from build123d import *

# Parameters (mm, degrees)
SKETCH_1_W                   = 25
SKETCH_1_H                   = 25
SKETCH_1_R                   = 1.5
EXTRUDE_1_DEPTH              = 7.65
SKETCH_2_R                   = 1.51
EXTRUDE_2_DEPTH              = 3
SKETCH_3_R                   = 7.5
CUT_EXTRUDE_1_DEPTH          = 5
SKETCH_4_R                   = 2.8
CUT_EXTRUDE_2_DEPTH          = 2
SKETCH_5_R                   = 1.55
CUT_EXTRUDE_3_DEPTH          = 2
SKETCH_6_W                   = 7.593154143
SKETCH_6_H                   = 30.65177665
CUT_EXTRUDE_4_DEPTH          = 30.911076544
EXTRUDE_START                = 0.5
SKETCH_7_R                   = 10
SKETCH_7_R_2                 = 7.5
EXTRUDE_3_DEPTH              = 0.5
FILLET_4_R                   = 2
HOLE_WIZARD_M2_1_D           = 1.6
HOLE_WIZARD_M2_1_CSINK_D     = 2.05
HOLE_WIZARD_M2_1_CSINK_ANGLE = 90


with BuildPart() as part:
    # 草图1 → 凸台-拉伸1 (new body)
    # profile 1 of 2: a face of its own
    with BuildSketch(Plane.XY):
        Rectangle(SKETCH_1_W, SKETCH_1_H)
        Circle(SKETCH_1_R, mode=Mode.SUBTRACT)
    # profile 2 of 2: a face of its own
    with BuildSketch(Plane.XY):
        Circle(SKETCH_1_R)
    extrude(amount=EXTRUDE_1_DEPTH)

    # 草图2 → 凸台-拉伸2 (add)
    with BuildSketch(Plane.XY.offset(7.65)):
        Circle(SKETCH_2_R)
    extrude(amount=EXTRUDE_2_DEPTH)

    # 草图3 → 切除-拉伸1 (cut)
    with BuildSketch(Plane(origin=(0, 0, 0), x_dir=(-1, 0, 0), z_dir=(0, 0, -1))):
        Circle(SKETCH_3_R)
    extrude(amount=-CUT_EXTRUDE_1_DEPTH, mode=Mode.SUBTRACT)

    # 草图4 → 切除-拉伸2 (cut)
    with BuildSketch(Plane.XY.offset(7.65)):
        with Locations((4.5, 0)):
            Circle(SKETCH_4_R)
        with Locations((-4.5, 0)):
            Circle(SKETCH_4_R)
    extrude(amount=-CUT_EXTRUDE_2_DEPTH, mode=Mode.SUBTRACT)

    # 草图5 → 切除-拉伸3 (cut)
    with BuildSketch(Plane.XY.offset(5.65)):
        with Locations((4.5, 0)):
            Circle(SKETCH_5_R)
        with Locations((-4.5, 0)):
            Circle(SKETCH_5_R)
    extrude(amount=-CUT_EXTRUDE_3_DEPTH, mode=Mode.SUBTRACT)

    # 草图6 → 切除-拉伸4 (cut, through all)
    with BuildSketch(Plane.ZY.offset(12.5)):
        with Locations((-2.946577072, 0.223328063)):
            Rectangle(SKETCH_6_W, SKETCH_6_H)
    extrude(amount=-CUT_EXTRUDE_4_DEPTH, mode=Mode.SUBTRACT)

    # 草图7 → 凸台-拉伸3 (add)
    with BuildSketch(Plane(origin=(0, 0, 0.85), x_dir=(-1, 0, 0), z_dir=(0, 0, -1)).offset(EXTRUDE_START)):
        with Locations(Location((0, 0, 0), (0, 0, 90))):
            Circle(SKETCH_7_R)
        Circle(SKETCH_7_R_2, mode=Mode.SUBTRACT)
    extrude(amount=-EXTRUDE_3_DEPTH)

    # 圆角4
    # the kernel refuses this fillet: 2 mm, written as the material it adds along each edge
    with BuildSketch(Plane(origin=(0, 0, 0.85), x_dir=(0, 1, 0), z_dir=(-1, 0, 0))) as fillet_4_piece_1:
        with BuildLine():
            CenterArc((11.322875656, 2), FILLET_4_R, 228.590377891, 41.409622109)
            Line((11.322875656, 0), (11.322875656, -0.04))
            Line((11.322875656, -0.04), (10, -0.04))
            Line((10, -0.04), (9.96, 0))
            ThreePointArc((9.96, 0), (9.96, 0.25), (9.973542487, 0.47))
            Line((9.973542487, 0.47), (10, 0.5))
        make_face()
    revolve(axis=Axis((0, 0, 0.85), (0, 0, -1)))

    # M2 螺纹孔1 (through all)
    with Locations(Plane.XY.offset(7.65)):
        with Locations((-10, 10), (10, 10), (-10, -10), (10, -10)):
            CounterSinkHole(HOLE_WIZARD_M2_1_D / 2, HOLE_WIZARD_M2_1_CSINK_D / 2, counter_sink_angle=HOLE_WIZARD_M2_1_CSINK_ANGLE)


solid = part.part
Read the model definition and answer for the solid it produces. Units are mm, in the model's axes. A direction names the side the tool comes from. Give positions to 0.01 mm unless a question says otherwise; leave off trailing zeros. Write each loop counter-clockwise with the first axis right and the second up, starting at its lowest first coordinate (ties: lowest second). Pieces come first, ordered by that corner, then holes. Notation, with made-up numbers: (71, 78) - (76, 78) arc R35 cw to (76, 111) - close; hole circle Ø7 at (-39.5, 37). An arc over 180 degrees is marked (long way). Use CSV: the item, a comma, the result in double quotes. Start each with the question number.
Item 1: Consider line 1 (Y direction, x = -10, z = 3.75); line 2 (X direction, y = -1.5, z = 6.5). Determine where each line is inside the solid, lowest interval first.
Item 2: The part is cut by section A-A, the plane x = 0. Give the vertices of the cut face in (y, z).
Item 3: The mould has two halves that part along Y. Classify faces 4 (the cylindrical face through (-0.197, 1.497, 9.129)), 5 (the flat face through (0, 12.5, 4)), 6 (the cylindrical face through (-9.896, -9.207, 4.091)): pulls with the +Y half, pulls with the -Y half, needs draft (parallel to the pull), parting line crosses it, or undercut.
Item 4: The part is cut by section C-C, the plane y = -0.5. Count the separate pieces of the cut face and the enclosed holes in it, and give its area (3 significant figures).
Item 5: The part is cut by section B-B, the plane z = 1.5. Give the vertices of the cut face in (x, y).
Item 6: Flat-ended cylindrical pins translate along their axes: P1, Ø4, axis at x = -4.5, y = 0, coming from the +Z side; P2, Ø10, axis at x = 5, y = -6.5, coming from the +Z side; P3, Ø5, axis at x = 4.5, y = 0, coming from the -Z side; P4, Ø1, axis at x = 10, y = -10, coming from the -Z side. Find the tip coordinate at first contact, or state that the pin passes through.
Item 7: For faces 1 (the flat face through (-12.5, 0, 4)), 2 (the flat face through (0, 0, 5)), 3 (the flat face through (6, -1, 5.65)), determine the directions among +Z, -Z, +X, -X, +Y, -Y from which every point of the face is accessible in a straight line to the end or side of a thin tool.
Item 8: The part is cut by section D-D, the plane z = 9. Give the vertices of the cut face in (x, y).
Taken from the geometry:
1,line 1,"-12.5 to -10.8, -9.2 to 9.2, 10.8 to 12.5"
1,line 2,"-12.5 to -6.86, -2.14 to 2.14, 6.86 to 12.5"
2,outline,"(-12.5, 0.85) - (-11.32, 0.85) arc R2 cw to (-10, 0.35) - (-7.5, 0.35) - (-7.5, 5) - (7.5, 5) - (7.5, 0.35) - (10, 0.35) arc R2 cw to (11.32, 0.85) - (12.5, 0.85) - (12.5, 7.65) - (1.51, 7.65) - (1.51, 10.65) - (-1.51, 10.65) - (-1.51, 7.65) - (-12.5, 7.65) - close"
3,face 4,"parting line crosses it"
3,face 5,"pulls with the +Y half"
3,face 6,"undercut"
4,separate pieces,"3"
4,enclosed holes,"0"
4,area,"93.5 mm2"
5,outline,"(-12.5, -12.5) - (12.5, -12.5) - (12.5, 12.5) - (-12.5, 12.5) - close; hole circle Ø1.6 at (-10, -10); hole circle Ø1.6 at (-10, 10); hole circle Ø15 at (0, 0); hole circle Ø1.6 at (10, -10); hole circle Ø1.6 at (10, 10)"
6,P1,"z = 5.65"
6,P2,"z = 7.65"
6,P3,"z = 5"
6,P4,"through"
7,face 1,"+Z, -Z, -X, +Y, -Y"
7,face 2,"-Z"
7,face 3,"+Z"
8,outline,"circle Ø3.02 at (0, 0)"
